The listing builds one solid part. Answer for the finished solid, in the listing's coordinates (mm). A direction names the side the tool comes from. Round coordinates to 2 decimals unless told otherwise and drop trailing zeros. Order: outer loops, then holes, each group sorted by start corner. A loop starts at its lowest first (then second) coordinate and runs counter-clockwise, first axis right, second up. Notation, with made-up numbers: (20.5, 13.5) - (37.5, 13.5) arc R16 ccw to (37.5, 40.5) - close; hole circle Ø7 at (24, 53.5). An arc over 180 degrees is marked (long way). Write item = value, one per line.
Autodesk Inventor part; units mm, degrees
ref_plane "YZ Plane" through (0, 0, 0) normal (1, 0, 0) x (0, 1, 0)
ref_plane "XZ Plane" through (0, 0, 0) normal (0, 1, 0) x (-1, 0, 0)
ref_plane "XY Plane" through (0, 0, 0) normal (0, 0, 1) x (1, 0, 0)
sketch "Sketch1" plane through (0, 0, 0) normal (0, 1, 0) x (-1, 0, 0)
  circle A0 centre (0, 0) radius 50
  dimension "d0" = 100
extrude "Extrusion1" add sketch "Sketch1" along normal blind 40
sketch "Sketch6" plane through (0, 0, 0) normal (0, -1, 0) x (1, 0, 0)
  circle A0 centre (0, 0) radius 5
  dimension "d36" = 10
extrude "Extrusion6" add sketch "Sketch6" along normal blind 60
thread "Thread1"
sketch "Sketch7" plane through (0, 40, 0) normal (0, 1, 0) x (1, 0, 0)
  line L0 (0, 0) -> (0, 50)
  circle A0 centre (0, 0) radius 5
  line L1 (-27.5, -47.6314) -> (-29.6651, -46.3814)
  line L2 (-29.6651, -46.3814) -> (-26.6651, -41.1852)
  line L3 (-22.3349, -43.6852) -> (-25.3349, -48.8814)
  line L4 (-25.3349, -48.8814) -> (-27.5, -47.6314)
  line L5 (-22.3349, -43.6852) -> (-26.6651, -41.1852)
  line L6 (-27.5, 47.6314) -> (-25.3349, 48.8814)
  line L7 (-25.3349, 48.8814) -> (-22.3349, 43.6852)
  line L8 (-22.3349, 43.6852) -> (-26.6651, 41.1852)
  line L9 (-26.6651, 41.1852) -> (-29.6651, 46.3814)
  line L10 (-29.6651, 46.3814) -> (-27.5, 47.6314)
  line L11 (55, 0) -> (55, 2.5)
  line L12 (55, 2.5) -> (49, 2.5)
  line L13 (49, 2.5) -> (49, -2.5)
  line L14 (49, -2.5) -> (55, -2.5)
  line L15 (55, -2.5) -> (55, 0)
  dimension "d52" = 5
  dimension "d55" = 6
  dimension "d58" = 2.5
  dimension "d60" = 5
extrude "Extrusion7" cut sketch "Sketch7" against normal blind 5 contours L1 L2 L5 L3 L4 | L6 L7 L8 L9 L10 | L15 L14 L13 L12 L11
sketch "Sketch8" plane through (-22.3349, 35, -43.6852) normal (-0.5, 0, -0.866) x (-0.866, 0, 0.5)
  line L0 (0, 5) -> (5, 5)
  line L1 (5, 5) -> (5, 0)
  line L2 (5, 5) -> (5, 0)
  line L3 (5, 0) -> (10, 0)
  line L4 (10, 0) -> (10, -5)
  line L5 (10, -5) -> (-5, -5)
  line L6 (-5, -5) -> (-5, 0)
  line L7 (-5, 0) -> (0, 0)
  line L8 (0, 0) -> (0, 5)
  line L9 (0, 5) -> (0, 0)
  point P0 (2.5, -35)
  dimension "d63" = 5
  dimension "d64" = 5
  dimension "d65" = 15
extrude "Extrusion8" cut sketch "Sketch8" along normal mid plane 60
sketch "Sketch9" plane through (49, 40, 2.5) normal (1, 0, 0) x (0, 0, -1)
  line L0 (5, 0) -> (0, 0)
  line L1 (0, 0) -> (5, 0)
  line L2 (0, 0) -> (0, -5)
  line L3 (0, -5) -> (0, 0)
  line L4 (0, -5) -> (-5, -5)
  line L5 (-5, -5) -> (-5, -10)
  line L6 (-5, -10) -> (10, -10)
  line L7 (10, -10) -> (10, -5)
  line L8 (10, -5) -> (5, -5)
  line L9 (5, -5) -> (5, 0)
  line L10 (5, 0) -> (5, -5)
  point P0 (2.5, -40)
  dimension "d68" = 5
  dimension "d69" = 5
  dimension "d70" = 15
extrude "Extrusion9" cut sketch "Sketch9" along normal mid plane 60
sketch "Sketch10" plane through (-26.6651, 35, 41.1852) normal (-0.5, 0, 0.866) x (0.866, 0, 0.5)
  line L0 (5, 5) -> (0, 5)
  line L1 (0, 5) -> (5, 5)
  line L2 (0, 5) -> (0, 0)
  line L3 (0, 0) -> (0, 5)
  line L4 (0, 0) -> (-5, 0)
  line L5 (-10.2045, 0) -> (-36.5614, 0)
  line L6 (-5, 0) -> (-5, -5)
  line L7 (-5, -5) -> (10, -5)
  line L8 (10, -5) -> (10, 0)
  line L9 (10, 0) -> (5, 0)
  line L10 (5, 0) -> (5, 5)
  point P0 (2.5, -35)
  dimension "d73" = 5
  dimension "d74" = 5
  dimension "d75" = 15
extrude "Extrusion10" cut sketch "Sketch10" along normal mid plane 60
sketch "Sketch11" plane through (0, 0, 0) normal (0, -1, 0) x (1, 0, 0)
  circle A0 centre (0, 25) radius 2.5
  point P0 (0, 0)
  dimension "d82" = 5
extrude "Extrusion11" add sketch "Sketch11" along normal blind 80
Q1. Find the intervals of material crossed by line 1 (Y direction, x = -30, z = -38.5); line 2 (Y direction, x = 0, z = 13.5); line 3 (Z direction, x = -34.5, y = 6), in increasing order. Write a range as from..to.
Model answer:
line_1 = 0..30, 35..40
line_2 = 0..40
line_3 = -36.19..36.19
Q2. Section C-C on y = -17 is taken. Determine the outline of the cut face in (x, z).
Model answer:
outline = circle Ø10 at (0, 0); circle Ø5 at (0, 25)
Q3. Determine the mould class of faces 4 (the face through (0, -80, 25)), 5 (the face through (34, 33, 7.5)) for opening direction Z: released by +Z, released by -Z, zero draft, split by the parting line, or undercut.
Model answer:
face_4 = zero draft
face_5 = undercut
Q4. For faces 1 (the face through (34, 38, 2.5)), 2 (the face through (-22, 35, 28)), 3 (the face through (34, 35, 5)), determine the directions among +Z, -Z, +X, -X, +Y, -Y from which every point of the face is accessible in a straight line to the end or side of a thin tool.
Model answer:
face_1 = +X, +Y
face_2 = none
face_3 = +X
Q5. Section A-A on x = 0 is taken. Determine the outline of the cut face in (y, z).
Model answer:
outline = (-80, 22.5) - (0, 22.5) - (0, 5) - (-60, 5) - (-60, -5) - (0, -5) - (0, -50) - (40, -50) - (40, 50) - (0, 50) - (0, 27.5) - (-80, 27.5) - close
Q6. Flat-ended cylindrical pins translate along their axes: P1, Ø22, axis at x = -12.5, z = 38, coming from the -Y side; P2, Ø8, axis at x = -3, y = 10, coming from the -Z side; P3, Ø5, axis at y = 1, z = 35.5, coming from the +X side; P4, Ø3, axis at y = -14, z = -7, coming from the +X side. Find the tip coordinate at first contact, or state that the pin passes through.
Model answer:
P1 = 0
P2 = -50
P3 = 37.56
P4 = through
Q7. Section B-B on z = 0 is taken. Determine the outline of the cut face in (x, y), then the cut area to 3 significant figures.
Model answer:
outline = (-50, 0) - (-5, 0) - (-5, -60) - (5, -60) - (5, 0) - (50, 0) - (50, 30) - (19, 30) - (19, 40) - (-50, 40) - close
area = 4,290 mm^2
Q8. Section D-D on x = 40 is taken. Determine the outline of the cut face in (y, z).
Model answer:
outline = (0, -30) - (40, -30) - (40, -2.5) - (35, -2.5) - (35, -7.5) - (30, -7.5) - (30, 7.5) - (35, 7.5) - (35, 2.5) - (40, 2.5) - (40, 30) - (0, 30) - close
